Design review of the part built by this model. Coordinates are the model's own, in mm. Face numbers are marked on the shaded views. Round coordinates to 2 decimals unless told otherwise and drop trailing zeros. Order: outer loops, then holes, each group sorted by start corner. A loop starts at its lowest first (then second) coordinate and runs counter-clockwise, first axis right, second up. Notation, with made-up numbers: (56.25, -10) - (84.25, -10) arc R15 ccw to (84.25, 6) - close; hole circle Ø3 at (-22.5, 59). An arc over 180 degrees is marked (long way). Write item = value, one per line.
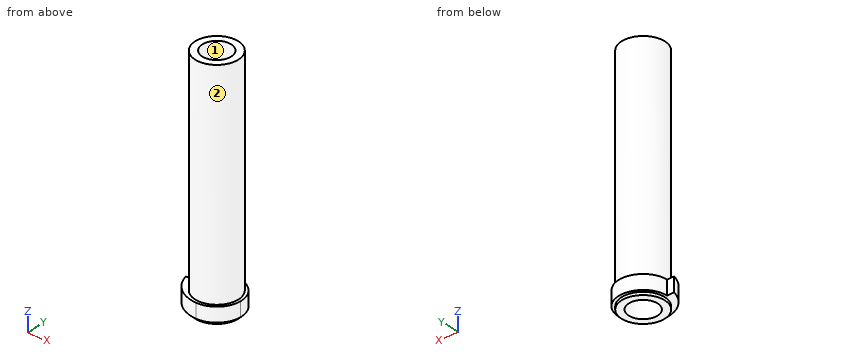
from build123d import *

# Parameters (mm, degrees)
F0_R      = 19.05
F1_DEPTH  = 205.74
F9_R      = 19.05
F10_DEPTH = 12.7
F11_R     = 12.7
F12_DEPTH = 254


with BuildPart() as f1:
    # F0 (on Top) → F1 (new body)
    with BuildSketch(Plane.XY):
        Circle(F0_R)
    extrude(amount=F1_DEPTH)

    # F9 (on offset) → F10 (join)
    with BuildSketch(Plane(origin=(0, 0, 2.54), x_dir=(1, 0, 0), z_dir=(0, 0, -1))):
        with BuildLine():
            ThreePointArc((-21.59, 0), (0, -21.59), (21.59, 0))
            ThreePointArc((21.59, 0), (15.266435, 15.266435), (0, 21.59))
            ThreePointArc((0, 21.59), (-15.266435, 15.266435), (-21.59, 0))
        make_face()
        Circle(F9_R, mode=Mode.SUBTRACT)
        with BuildLine():
            ThreePointArc((-21.59, 0), (-15.266435, 15.266435), (0, 21.59))
            ThreePointArc((0, 21.59), (-17.654827, 15.5636), (-27.94, 0))
            Line((-27.94, 0), (-21.59, 0))
        make_face()
    extrude(amount=-F10_DEPTH)

    # F11 (on face) → F12 (cut)
    with BuildSketch(Plane(origin=(0, 0, 0), x_dir=(1, 0, 0), z_dir=(0, 0, -1))):
        Circle(F11_R)
    extrude(amount=-F12_DEPTH, mode=Mode.SUBTRACT)


solid = f1.part
Item 1: For line 1 along X through (y, z) = (0, 59); line 2 along Z through (x, y) = (16, -12), list the stretches that pass through material, from the lowest coordinate up. Write a range as [from, to].
Data:
line_1 = [-19.05, -12.7], [12.7, 19.05]
line_2 = [2.54, 15.24]
Item 2: Insertion check: P1, Ø4, axis at y = -9.5, z = 157, coming from the -X side; P2, Ø1.5, axis at x = 8, z = 95, coming from the +Y side; P3, Ø1.9, axis at x = -26, z = 11.5, coming from the +Y side; P4, Ø10, axis at x = 16.5, y = 15.5, coming from the +Z side. Each pin has a flat end and moves straight along its axis. Give the tip position at first contact, or say it passes through.
Data:
P1 = -17.51
P2 = 17.62
P3 = 0
P4 = 205.74
Item 3: Take a section at A-A, the plane y = 4. State the section outline as (x, z) points, and give its area (3 significant figures).
Data:
outline = (-21.22, 2.54) - (-18.63, 2.54) - (-18.63, 0) - (-12.05, 0) - (-12.05, 205.74) - (-18.63, 205.74) - (-18.63, 15.24) - (-21.22, 15.24) - close; (12.05, 0) - (18.63, 0) - (18.63, 2.54) - (21.22, 2.54) - (21.22, 15.24) - (18.63, 15.24) - (18.63, 205.74) - (12.05, 205.74) - close
area = 2,770 mm2
Item 4: Take a section at D-D, the plane x = -16. State the section outline as (y, z) points.
Data:
outline = (-16.75, 2.54) - (-10.34, 2.54) - (-10.34, 0) - (10.34, 0) - (10.34, 2.54) - (14.5, 2.54) - (14.5, 15.24) - (10.34, 15.24) - (10.34, 205.74) - (-10.34, 205.74) - (-10.34, 15.24) - (-16.75, 15.24) - close
Item 5: The part is to be moulded in two halves that separate along Y. For the marked faces 1 and 2, say which applies: +Y half, -Y half, draft (parallel to the pull), parting line (faces both ways), or undercut.
Data:
face_1 = undercut
face_2 = parting line
Item 6: Take a section at B-B, the plane x = -7. State the section outline as (y, z) points.
Data:
outline = (-20.73, 2.54) - (-17.72, 2.54) - (-17.72, 0) - (-10.6, 0) - (-10.6, 205.74) - (-17.72, 205.74) - (-17.72, 15.24) - (-20.73, 15.24) - close; (10.6, 0) - (17.72, 0) - (17.72, 2.54) - (20.42, 2.54) - (20.42, 15.24) - (17.72, 15.24) - (17.72, 205.74) - (10.6, 205.74) - close
Item 7: Take a section at C-C, the plane z = 187. State the section outline as (x, y) points.
Data:
outline = circle Ø38.1 at (0, 0); hole circle Ø25.4 at (0, 0)
